from build123d import *

# Parameters (mm, degrees)
F1_DEPTH = 62
F2_R     = 1.65
F3_DEPTH = 25
F4_R     = 2
F4_R_2   = 2.75
F5_DEPTH = 25


with BuildPart() as f1:
    # F0 (on Front) → F1 (new body)
    with BuildSketch(Plane.XZ):
        with BuildLine():
            ThreePointArc((2, 12.440257), (0, -12.6), (-2, 12.440257))
            Line((-2, 12.440257), (-2, 28))
            Line((-2, 28), (-7, 28))
            Line((-7, 28), (-7, 14.498621))
            ThreePointArc((-7, 14.498621), (-15.952875, 2.171583), (-10.620734, -12.1))
            Line((-10.620734, -12.1), (-21.1, -12.1))
            Line((-21.1, -12.1), (-21.1, -16.1))
            Line((-21.1, -16.1), (0, -16.1))
            Line((0, -16.1), (21.1, -16.1))
            Line((21.1, -16.1), (21.1, -12.1))
            Line((21.1, -12.1), (10.620734, -12.1))
            ThreePointArc((10.620734, -12.1), (15.952875, 2.171583), (7, 14.498621))
            Line((7, 14.498621), (7, 28))
            Line((7, 28), (2, 28))
            Line((2, 28), (2, 12.440257))
        make_face()
    extrude(amount=F1_DEPTH)

    # F2 (on face) → F3 (cut)
    with BuildSketch(Plane.XY.offset(-12.1)):
        with Locations((15.5, -15.5)):
            Circle(F2_R)
        with Locations((15.5, -46.5)):
            Circle(F2_R)
        with Locations((-15.5, -15.5)):
            Circle(F2_R)
        with Locations((-15.5, -46.5)):
            Circle(F2_R)
    extrude(amount=-F3_DEPTH, mode=Mode.SUBTRACT)

    # F4 (on face) → F5 (cut)
    with BuildSketch(Plane.XY.offset(-12.1)):
        with Locations((15.5, -46.5)):
            Circle(F4_R)
        with Locations((15.5, -15.5)):
            Circle(F4_R_2)
    extrude(amount=F5_DEPTH, mode=Mode.SUBTRACT)


solid = f1.part
Geometry check sheet. Reference: the model listing, model coordinates, mm. A direction names the side the tool comes from. Round coordinates to 2 decimals unless told otherwise and drop trailing zeros. Write each loop counter-clockwise with the first axis right and the second up, starting at its lowest first coordinate (ties: lowest second). Pieces come first, ordered by that corner, then holes. Notation, with made-up numbers: (39.25, 47) -> (62.25, 47) arc R11 ccw to (62.25, 53) -> close; hole circle Ø4 at (3, 14.5). An arc over 180 degrees is marked (long way). One line per item, written item: value. Start each with the question number.
(1) Go/stop test with flat-tipped pins: pin 1 Ø3 at (x, y) = (-15.5, -46.5) entering from -Z; pin 2 Ø2 at (x, y) = (0.5, -41.5) entering from +Z; pin 3 Ø5 at (y, z) = (-41, 16) entering from -X; pin 4 Ø2 at (x, y) = (15.5, -15.5) entering from +Z. Record where each tip stops, or that it passes through.
(2) Access from +Z, -Z, +X, -X, +Y, -Y to the whole of each face (thin tool, end or side, straight path). Record for faces 4 (the flat face through (-7, -31, 21)), 5 (the flat face through (7, -31, 21)), 6 (the flat face through (-2, -31, 20)).
(3) Cross-section at C-C, the plane x = 11.5. Record the cut outline in (y, z), and give its area (3 significant figures).
(4) Cross-section at B-B, the plane z = 6. Record the cut outline in (x, y), and give its area (3 significant figures).
(5) Draft check along X on faces 1 (the flat face through (0, -31, -16.1)), 2 (the cylindrical face through (0.53, -30.57, -12.59)), 3 (the flat face through (21.1, -31, -14)). Enter one of: +X half, -X half, draft (parallel to the pull), parting line (faces both ways), or undercut.
(6) Scan lines: line 1 (Y direction, x = 15.5, z = -13.95); line 2 (X direction, y = -36, z = 23); line 3 (Y direction, x = 15, z = -1). Record each from-to range of solid material in increasing order. Write a range as [from, to].
(7) Cross-section at A-A, the plane y = -15.5. Record the cut outline in (x, z), and give its area (3 significant figures).
(8) Cross-section at D-D, the plane y = -5. Record the cut outline in (x, z).
Answer:
1. pin 1: z = -7.95
1. pin 2: z = -12.51
1. pin 3: x = -8.77
1. pin 4: through
2. face 4: +Z, -X, +Y, -Y
2. face 5: +Z, +X, +Y, -Y
2. face 6: +Z, +Y, -Y
3. outline: (-62, -16.1) -> (0, -16.1) -> (0, -12.1) -> (-62, -12.1) -> close; (-62, -11.27) -> (0, -11.27) -> (0, -5.15) -> (-62, -5.15) -> close; (-62, 5.15) -> (0, 5.15) -> (0, 11.27) -> (-62, 11.27) -> close
3. area: 1,010 mm²
4. outline: (-14.94, -62) -> (-11.08, -62) -> (-11.08, 0) -> (-14.94, 0) -> close; (11.08, -62) -> (14.94, -62) -> (14.94, -48.42) arc R2 cw to (14.94, -44.58) -> (14.94, -18.19) arc R2.75 cw to (14.94, -12.81) -> (14.94, 0) -> (11.08, 0) -> close
4. area: 466 mm²
5. face 1: draft
5. face 2: undercut
5. face 3: +X half
6. line 1: [-62, -48.15], [-44.85, -17.15], [-13.85, 0]
6. line 2: [-7, -2], [2, 7]
6. line 3: [-62, -48.44], [-44.56, -18.2], [-12.8, 0]
7. outline: (-21.1, -16.1) -> (-17.15, -16.1) -> (-17.15, -12.1) -> (-21.1, -12.1) -> close; (-13.85, -16.1) -> (13.85, -16.1) -> (13.85, -12.1) -> (10.62, -12.1) arc R16.1 ccw to (12.75, -9.83) -> (12.75, 9.83) arc R16.1 ccw to (7, 14.5) -> (7, 28) -> (2, 28) -> (2, 12.44) arc R12.6 cw (long way) to (-2, 12.44) -> (-2, 28) -> (-7, 28) -> (-7, 14.5) arc R16.1 ccw to (-10.62, -12.1) -> (-13.85, -12.1) -> close; (17.15, -16.1) -> (21.1, -16.1) -> (21.1, -12.1) -> (17.15, -12.1) -> close
7. area: 467 mm²
8. outline: (-21.1, -16.1) -> (21.1, -16.1) -> (21.1, -12.1) -> (10.62, -12.1) arc R16.1 ccw to (7, 14.5) -> (7, 28) -> (2, 28) -> (2, 12.44) arc R12.6 cw (long way) to (-2, 12.44) -> (-2, 28) -> (-7, 28) -> (-7, 14.5) arc R16.1 ccw to (-10.62, -12.1) -> (-21.1, -12.1) -> close
